Print and shaded views of the part. All mm, measured from the part's lowest x, y and z. A direction names the side the tool comes from. Round coordinates to 2 decimals unless told otherwise and drop trailing zeros. Loops run counter-clockwise (first coordinate to the right, second up) from the corner with the lowest first, then second, coordinate; pieces in that order, holes last. Notation, with made-up numbers: (0.5, 12) - (11.5, 12) arc R21 cw to (11.5, 46) - close; hole circle Ø10 at (15.25, -26.75). An arc over 180 degrees is marked (long way). Use one line per item in the form item = value.
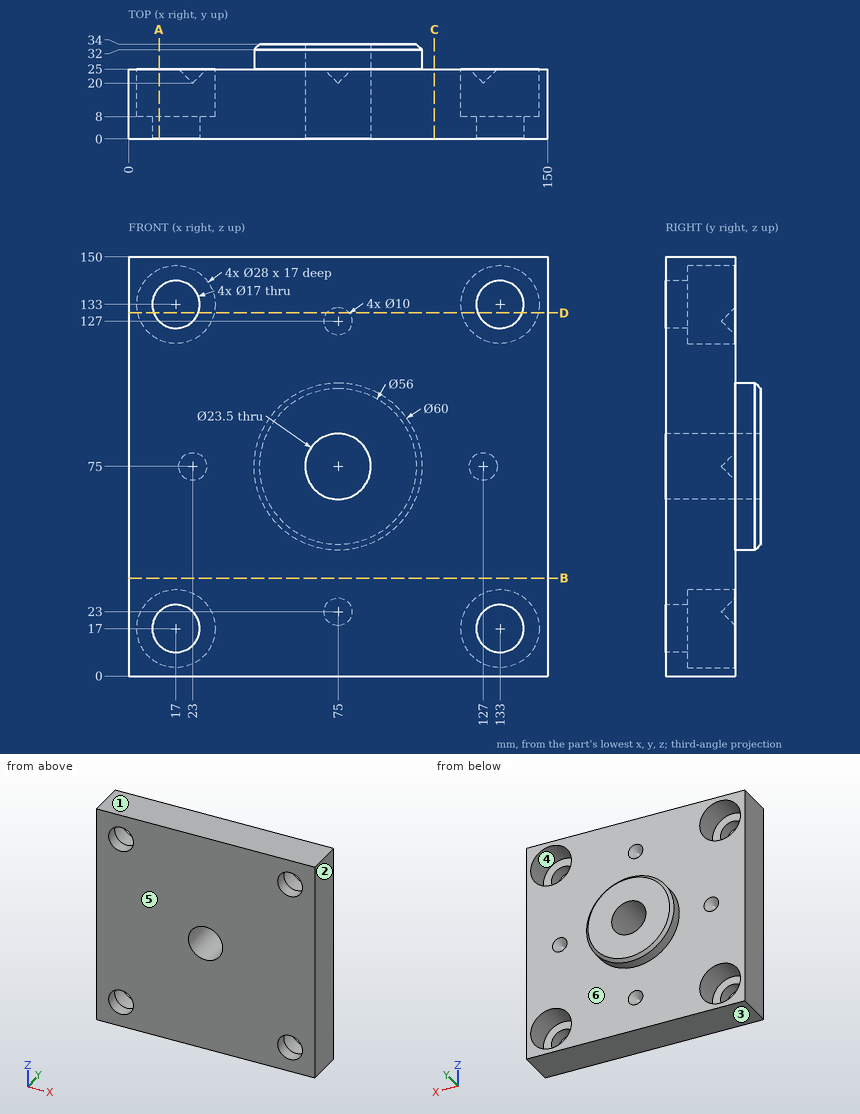
1. Cut at D-D, the plane z = 130. Give the number of separate pieces and of enclosed holes in the cut face, plus the area to 3 significant figures.
Geometry check:
separate_pieces = 3
enclosed_holes = 0
area = 2,560 mm^2
2. Pull direction Z, two halves, no side cores. Call the marked faces 1, 2, 3 and 4: +Z half, -Z half, draft (parallel to the pull), parting line (faces both ways), or undercut.
Geometry check:
face_1 = +Z half
face_2 = draft
face_3 = -Z half
face_4 = undercut
3. Cut at C-C, the plane x = 109.5. Give the cut face in (y, z).
Geometry check:
outline = (0, 0) - (25, 0) - (25, 150) - (0, 150) - close
4. Wall check: probe 1 along Z at (x, y) = (133, 2); probe 2 along Z at (x, y) = (133, 15). Give the ranges that are in metal, low to high.
Geometry check:
probe_1 = 0 to 8.5, 25.5 to 124.5, 141.5 to 150
probe_2 = 0 to 3, 31 to 119, 147 to 150
5. Cut at B-B, the plane z = 35. Give the cut face in (x, y).
Geometry check:
outline = (0, 0) - (150, 0) - (150, 25) - (0, 25) - close
6. Tool access for the marked faces 5 and 6: list every direction of +Z, -Z, +X, -X, +Y, -Y with a clear straight run to the whole face (end or side of a thin tool).
Geometry check:
face_5 = +Z, -Z, +X, -X, -Y
face_6 = +Y
7. Cut at A-A, the plane x = 11. Give the cut face in (y, z).
Geometry check:
outline = (0, 0) - (25, 0) - (25, 4.35) - (8, 4.35) - (8, 10.98) - (0, 10.98) - close; (0, 23.02) - (8, 23.02) - (8, 29.65) - (25, 29.65) - (25, 120.35) - (8, 120.35) - (8, 126.98) - (0, 126.98) - close; (0, 139.02) - (8, 139.02) - (8, 145.65) - (25, 145.65) - (25, 150) - (0, 150) - close
8. Flat gauge pins, fed straight in: pin 1 (15.5 mm diameter, centred on x = 17, z = 17, fed in from +Y); pin 2 (4 mm diameter, centred on x = 30.5, z = 75.5, fed in from +Y); pin 3 (14 mm diameter, centred on x = 21.5, z = 129.5, fed in from +Y). Where does each tip first touch, or does it go through?
Geometry check:
pin_1 = through
pin_2 = 25
pin_3 = 8
